Geometry: final body of the model. Coordinates: model frame, mm. Face numbers are marked on the shaded views. A direction names the side the tool comes from. Round coordinates to 2 decimals unless told otherwise and drop trailing zeros. Loops run counter-clockwise (first coordinate to the right, second up) from the corner with the lowest first, then second, coordinate; pieces in that order, holes last. Notation, with made-up numbers: M 39,54.5 L 51,54.5 A7 ccw 51,62.5 Z; hole C 62,39.5 d7. An arc over 180 degrees is marked long. Write each question's results on one line, items separated by ' | '.
```python
from build123d import *

# Parameters (mm, degrees)
SKETCH_3_W          = 8
SKETCH_3_H          = 15
EXTRUDE_1_DEPTH     = 14
SKETCH_4_R          = 1.5
CUT_EXTRUDE_1_DEPTH = 10
FILLET_1_R          = 1


with BuildPart() as part:
    # ｽｹｯﾁ1 → 回転2 (revolve)
    with BuildSketch(Plane.XY):
        with BuildLine():
            Line((-19.5, 10.435516279), (19.5, 10.435516279))
            ThreePointArc((19.5, 10.435516279), (23.540844472, 5.898092912), (25, 0))
            Line((25, 0), (-25, 0))
            ThreePointArc((-25, 0), (-23.540844472, 5.898092912), (-19.5, 10.435516279))
        make_face()
    revolve(axis=Axis((-19.5, 0, 0), (1, 0, 0)))

    # ｽｹｯﾁ3 → ﾎﾞｽ - 押し出し1 (add)
    with BuildSketch(Plane(origin=(0, 0, 0), x_dir=(1, 0, 0), z_dir=(0, 1, 0))):
        with Locations((-11.5, 0)):
            Rectangle(SKETCH_3_W, SKETCH_3_H)
        with Locations((11.5, 0)):
            Rectangle(SKETCH_3_W, SKETCH_3_H)
    extrude(amount=-EXTRUDE_1_DEPTH)

    # ｽｹｯﾁ4 → ｶｯﾄ - 押し出し1 (cut)
    with BuildSketch(Plane(origin=(0, -14, 0), x_dir=(-1, 0, 0), z_dir=(0, -1, 0))):
        with Locations(Location((-11.5, 0, 0), (0, 0, 90))):
            Circle(SKETCH_4_R)
        with Locations(Location((11.5, 0, 0), (0, 0, 90))):
            Circle(SKETCH_4_R)
    extrude(amount=-CUT_EXTRUDE_1_DEPTH, mode=Mode.SUBTRACT)

    # ﾌｨﾚｯﾄ1
    fillet_1_edges = [part.edges().sort_by_distance(p)[0] for p in [
        (-19.5, -10.435516279, 0),
        (19.5, -10.435516279, 0),
    ]]
    fillet(fillet_1_edges, radius=FILLET_1_R)


solid = part.part
```
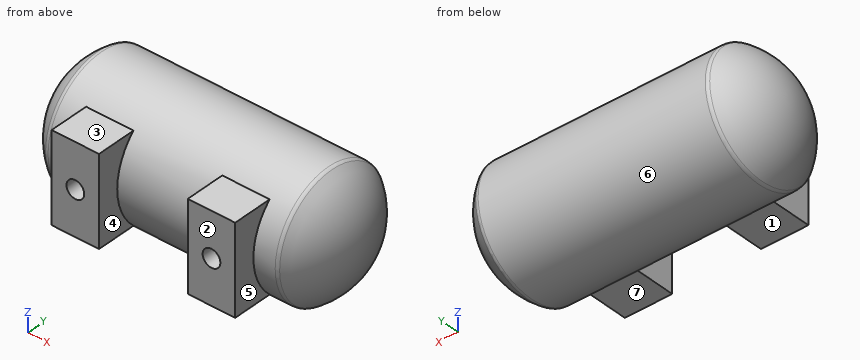
1. Draft query along X for the marked faces 4, 5, 6 and 7. Return one class per face: pulls with the +X half, pulls with the -X half, needs draft (parallel to the pull), parting line crosses it, or undercut.
Answer key:
face 4: undercut | face 5: pulls with the +X half | face 6: undercut | face 7: needs draft
2. Ray query, probe 1 along X at (y, z) = (-11.75, 0); probe 2 along X at (y, z) = (-9.25, -5.75); probe 3 along X at (y, z) = (-6.25, 0). Return the intervals inside material, ascending.
Answer key:
probe 1: x = -15.5 to -13, -10 to -7.5, 7.5 to 10, 13 to 15.5 | probe 2: x = -15.5 to -7.5, 7.5 to 15.5 | probe 3: x = -23.35 to -13, -10 to 10, 13 to 23.35
3. Section A-A (x = 11.5). Output: boundary loops of the cut face in (y, z), then the cut area to 3 significant figures.
Answer key:
outline: M -14,-7.5 L -7.26,-7.5 A10.44 ccw long -7.26,7.5 L -14,7.5 L -14,1.5 L -4,1.5 L -4,-1.5 L -14,-1.5 Z | area: 380 mm²
4. Pin query (flat end, axial travel): P1, Ø5.5, axis at x = 12, y = -11, coming from the -Z side; P2, Ø4, axis at y = -5.5, z = 3.5, coming from the -X side; P3, Ø3, axis at x = 18, y = 4.5, coming from the -Z side (3 decimals). Return the tip coordinate at first contact, or that it passes through.
Answer key:
P1: stops at z = -7.5 | P2: stops at x = -24.17 | P3: stops at z = -9.995
5. Access query for the marked faces 1, 2 and 3. Directions: +Z, -Z, +X, -X, +Y, -Y. A direction counts if a zero-diameter tool reaches every point of the face in a straight line with its end or side. Return the directions, or none.
Answer key:
face 1: -Z, +X, -X, -Y | face 2: +Z, -Z, +X, -X, -Y | face 3: +Z, +X, -X, -Y
6. Section B-B (x = -16). Output: boundary loops of the cut face in (y, z), then the cut area to 3 significant figures.
Answer key:
outline: C 0,0 d20.87 | area: 342 mm²
